```python
from build123d import *

# Parameters (mm, degrees)
BOSS_EXTRUDE1_DEPTH      = 3
BOSS_EXTRUDE1_DEPTH_BACK = 3
BOSS_EXTRUDE2_DEPTH      = 5.6
SKETCH3_R                = 2
BOSS_EXTRUDE3_DEPTH      = 10


with BuildPart() as part:
    # Sketch1 → Boss-Extrude1 (new, two sides: drawn at the far end of the back side and taken through both)
    with BuildSketch(Plane(origin=(0, 0, 0), x_dir=(1, 0, 0), z_dir=(0, 1, 0)).offset(-BOSS_EXTRUDE1_DEPTH_BACK)):
        with BuildLine():
            Line((-12.55, 8), (10.05, 8))
            ThreePointArc((10.05, 8), (11.817766953, 7.267766953), (12.55, 5.5))
            Line((12.55, 5.5), (12.55, -5.5))
            ThreePointArc((12.55, -5.5), (11.817766953, -7.267766953), (10.05, -8))
            Line((10.05, -8), (-12.55, -8))
            Line((-12.55, -8), (-12.55, 8))
        make_face()
    extrude(amount=BOSS_EXTRUDE1_DEPTH + BOSS_EXTRUDE1_DEPTH_BACK)

    # Sketch2 → Boss-Extrude2 (add)
    with BuildSketch(Plane.ZY.offset(12.55)):
        with BuildLine():
            Line((6.3, 1.044645313), (6.3, 1.15))
            Line((6.3, 1.15), (-6.3, 1.15))
            Line((-6.3, 1.15), (-6.3, -1.15))
            Line((-6.3, -1.15), (-2, -1.15))
            Line((-2, -1.15), (-2, -0.605330086))
            ThreePointArc((-2, -0.605330086), (-1.52157966, 0.110676552), (-0.676992245, -0.05732233))
            Line((-0.676992245, -0.05732233), (0.064213562, -0.798528137))
            ThreePointArc((0.064213562, -0.798528137), (0.453521581, -1.058655439), (0.9127417, -1.15))
            Line((0.9127417, -1.15), (4.105354687, -1.15))
            ThreePointArc((4.105354687, -1.15), (4.564574806, -1.058655439), (4.953882825, -0.798528137))
            Line((4.953882825, -0.798528137), (5.948528137, 0.196117175))
            ThreePointArc((5.948528137, 0.196117175), (6.208655439, 0.585425194), (6.3, 1.044645313))
        make_face()
        with BuildLine():
            Line((4.812461468, -0.657106781), (5.807106781, 0.337538532))
            ThreePointArc((5.807106781, 0.337538532), (6.004712185, 0.618622002), (6.095511057, 0.95))
            Line((6.095511057, 0.95), (-6.1, 0.95))
            Line((-6.1, 0.95), (-6.1, -0.95))
            Line((-6.1, -0.95), (-2.2, -0.95))
            Line((-2.2, -0.95), (-2.2, -0.605330086))
            ThreePointArc((-2.2, -0.605330086), (-1.598116347, 0.295452458), (-0.535570888, 0.084099026))
            Line((-0.535570888, 0.084099026), (0.205634919, -0.657106781))
            ThreePointArc((0.205634919, -0.657106781), (0.530058267, -0.873879533), (0.9127417, -0.95))
            Line((0.9127417, -0.95), (4.105354687, -0.95))
            ThreePointArc((4.105354687, -0.95), (4.48803812, -0.873879533), (4.812461468, -0.657106781))
        make_face(mode=Mode.SUBTRACT)
    extrude(amount=BOSS_EXTRUDE2_DEPTH)

    # Sketch3 → Boss-Extrude3 (add)
    with BuildSketch(Plane(origin=(12.55, 0, 0), x_dir=(0, 0, -1), z_dir=(1, 0, 0))):
        Circle(SKETCH3_R)
    extrude(amount=BOSS_EXTRUDE3_DEPTH)


solid = part.part
```
CAD build for the part. Positions are in the model's coordinates, mm. A direction names the side the tool comes from. Round coordinates to 2 decimals unless told otherwise and drop trailing zeros. Loops run counter-clockwise (first coordinate to the right, second up) from the corner with the lowest first, then second, coordinate; pieces in that order, holes last. Notation, with made-up numbers: (25, 52.25) - (79, 52.25) arc R28 ccw to (79, 85.25) - close; hole circle Ø1 at (-18.75, 48.5). An arc over 180 degrees is marked (long way). Return JSON: item names as keys, results as strings. Group by question number.
Q1. Band-saw the part on B-B on x = 17. Give the cut face in (y, z), plus the area to 3 significant figures.
Q2. Band-saw the part on C-C on z = -1.25. Give the cut face in (x, y), plus the area to 3 significant figures.
Q3. Two-plate mould, pull along Z, no slides. Class faces 4 (the face through (0, -3, 0)), 5 (the face through (-12.55, 0, 0)), 6 (the face through (-15.31, -0.31, 5.44)): +Z half, -Z half, draft (parallel to the pull), parting line (faces both ways), or undercut.
Q4. Tool access for faces 1 (the face through (-15, 0, -6.3)), 2 (the face through (-15, -1.15, -4)), 3 (the face through (17, -2, 0)): list every direction of +Z, -Z, +X, -X, +Y, -Y with a clear straight run to the whole face (end or side of a thin tool).
Q5. Flat gauge pins, fed straight in: pin 1 Ø1.2 at (x, z) = (-14.5, -5) entering from +Y; pin 2 Ø1.8 at (x, y) = (-16, -0.5) entering from -Z; pin 3 Ø1 at (x, y) = (-14, -0.5) entering from +Z; pin 4 Ø1.5 at (x, y) = (-13.5, -2) entering from -Z. Where does each tip first touch, or does it go through?
Q6. Band-saw the part on A-A on z = -3.5. Give the cut face in (x, y), plus the area to 3 significant figures.
Q7. Drill centre lines: line 1 along X through (y, z) = (-1.4, -1.5); line 2 along X through (y, z) = (-0.15, 0.25); line 3 along Z through (x, y) = (13.5, -1.3). Where is each one in solid material? Low to high. Write a range as [from, to].
Q8. Band-saw the part on D-D on z = 6.75. Give the cut face in (x, y), plus the area to 3 significant figures.
Solutions:
{
 "1": {"outline": "circle Ø4 at (0, 0)", "area": "12.6 mm^2"},
 "2": {"outline": "(-18.15, 0.17) - (-12.55, 0.17) - (-12.55, -3) - (12.55, -3) - (12.55, -1.56) - (22.55, -1.56) - (22.55, 1.56) - (12.55, 1.56) - (12.55, 3) - (-12.55, 3) - (-12.55, 1.15) - (-18.15, 1.15) - (-18.15, 0.95) - (-12.55, 0.95) - (-12.55, 0.37) - (-18.15, 0.37) - close", "area": "184 mm^2"},
 "3": {"face 4": "draft", "face 5": "undercut", "face 6": "+Z half"},
 "4": {"face 1": "-Z, -X, +Y, -Y", "face 2": "+Z, -Z, -X, -Y", "face 3": "+X"},
 "5": {"pin 1": "stops at y = 1.15", "pin 2": "stops at z = -6.3", "pin 3": "stops at z = 5.75", "pin 4": "passes through"},
 "6": {"outline": "(-18.15, -1.15) - (-12.55, -1.15) - (-12.55, -3) - (12.55, -3) - (12.55, 3) - (-12.55, 3) - (-12.55, 1.15) - (-18.15, 1.15) - (-18.15, 0.95) - (-12.55, 0.95) - (-12.55, -0.95) - (-18.15, -0.95) - close", "area": "153 mm^2"},
 "7": {"line 1": "x = [-12.55, 12.55]", "line 2": "x = [-12.55, 22.55]", "line 3": "z = [-1.52, 1.52]"},
 "8": {"outline": "(-12.55, -3) - (12.22, -3) - (12.22, 3) - (-12.55, 3) - close", "area": "149 mm^2"}
}
